Can you work these out from the model? Positions are in its coordinate system, mm. Round coordinates to 2 decimals unless told otherwise and drop trailing zeros. Loops run counter-clockwise (first coordinate to the right, second up) from the corner with the lowest first, then second, coordinate; pieces in that order, holes last. Notation, with made-up numbers: (-32.75, 82.25) -> (-23.75, 82.25) arc R25 ccw to (-23.75, 105.25) -> close; hole circle Ø8 at (1, 62.25). An arc over 180 degrees is marked (long way). Answer as a JSON object with one key per item and string values.
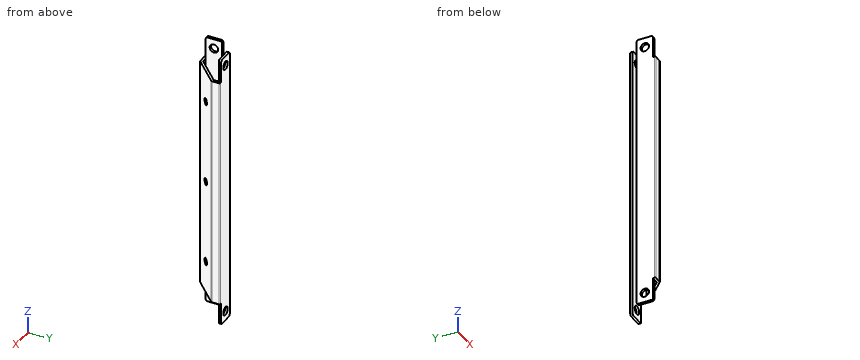
```python
from build123d import *

# Parameters (mm, degrees)
F1_DEPTH = 172.5
F3_DEPTH = 28
F4_R     = 4.25
F5_DEPTH = 25
F6_R     = 5.25
F7_DEPTH = 25
F8_R     = 5.25
F9_DEPTH = 25
F10_R    = 2
F11_R    = 0.5
F12_R    = 1


# Not quite as in the source:
# - a pattern or mirror of a feature is missing from the dataset's text; its kind, count and spacing are read off the source's solid


with BuildPart() as f1:
    # F0 (on Top) → F1 (new body, symmetric)
    with BuildSketch(Plane.XY):
        Polygon((-19.75, 3.25), (-19.75, -19.75), (-9.25, -19.75), (19.75, 9.25), (19.75, 19.75), (-3.25, 19.75), (-3.25, 16.75), (16.75, 16.75), (16.75, 10.4926406871), (-10.4926406871, -16.75), (-16.75, -16.75), (-16.75, 3.25), align=None)
    extrude(amount=F1_DEPTH, both=True)

    # F2 (on face) → F3 (cut)
    with BuildSketch(Plane.XY.offset(172.5)):
        Polygon((-10.4926406871, -16.75), (-16.75, -16.75), (-19.75, -16.75), (-19.75, -19.75), (-9.25, -19.75), (19.75, 9.25), (19.75, 19.75), (16.75, 19.75), (16.75, 16.75), (16.75, 10.4926406871), align=None)
    f3 = extrude(amount=-F3_DEPTH, mode=Mode.SUBTRACT)

    # F3_copies: F3 across plane
    add(f3.mirror(Plane(origin=(0, 0, 0), x_dir=(-1, 0, 0), z_dir=(0, 0, -1))), mode=Mode.SUBTRACT)

    # F4 (on face) → F5 (cut)
    with BuildSketch(Plane(origin=(5.25, -5.25, 0), x_dir=(0.7071067812, 0.7071067812, 0), z_dir=(0.7071067812, -0.7071067812, 0))):
        with Locations((0, 104.5)):
            Circle(F4_R)
        with Locations((0, -104.5)):
            Circle(F4_R)
        Circle(F4_R)
    extrude(amount=-F5_DEPTH, mode=Mode.SUBTRACT)

    # F6 (on face) → F7 (cut)
    with BuildSketch(Plane.YZ.offset(-16.75)):
        with Locations((-6.75, 160.5)):
            Circle(F6_R)
        with Locations((-6.75, -160.5)):
            Circle(F6_R)
    extrude(amount=-F7_DEPTH, mode=Mode.SUBTRACT)

    # F8 (on face) → F9 (cut)
    with BuildSketch(Plane.XZ.offset(-16.75)):
        with Locations((6.75, 160.5)):
            Circle(F8_R)
        with Locations((6.75, -160.5)):
            Circle(F8_R)
    extrude(amount=-F9_DEPTH, mode=Mode.SUBTRACT)

    # F10
    f10_edges = [f1.edges().sort_by_distance(p)[0] for p in [
        (-9.25, -19.75, 0),
        (19.75, 9.25, 0),
        (16.75, 18.25, 172.5),
        (-3.25, 18.25, 172.5),
        (-18.25, 3.25, 172.5),
        (-18.25, -16.75, 172.5),
        (-18.25, 3.25, -172.5),
        (-3.25, 18.25, -172.5),
        (-18.25, -16.75, -172.5),
        (16.75, 18.25, -172.5),
    ]]
    fillet(f10_edges, radius=F10_R)

    # F11
    f11_edges = [f1.edges().sort_by_distance(p)[0] for p in [
        (-10.492641, -16.75, 0),
        (16.75, 10.492641, 0),
    ]]
    fillet(f11_edges, radius=F11_R)

    # F12
    f12_edges = [f1.edges().sort_by_distance(p)[0] for p in [
        (-19.75, -19.75, 0),
        (19.75, 19.75, 0),
    ]]
    fillet(f12_edges, radius=F12_R)


solid = f1.part
```
Q1. I'm going to push flat-ended pins straight in: pin 1 (6 mm diameter, centred on x = 8, z = 80, fed in from -Y); pin 2 (2.5 mm diameter, centred on y = 17.5, z = 152.5, fed in from +X); pin 3 (1.5 mm diameter, centred on y = 19, z = 32, fed in from -X). Where does each tip first touch, or does it pass through?
Determined:
{"pin 1": "y = -5.5", "pin 2": "x = 16.75", "pin 3": "x = -3.25"}
Q2. I want a section at A-A, the plane z = -160.5. Write out the boundary of the cut face in (x, y), then the cut area to 3 significant figures.
Determined:
{"outline": "(-19.75, -16.75) -> (-16.75, -16.75) -> (-16.75, -12) -> (-19.75, -12) -> close; (-19.75, -1.5) -> (-16.75, -1.5) -> (-16.75, 3.25) -> (-19.75, 3.25) -> close; (-3.25, 16.75) -> (1.5, 16.75) -> (1.5, 19.75) -> (-3.25, 19.75) -> close; (12, 16.75) -> (16.75, 16.75) -> (16.75, 19.75) -> (12, 19.75) -> close", "area": "57.0 mm²"}
Q3. I want a section at B-B, the plane z = -32. Write out the boundary of the cut face in (x, y), then the cut area to 3 significant figures.
Determined:
{"outline": "(-19.75, -18.75) arc R1 ccw to (-18.75, -19.75) -> (-10.08, -19.75) arc R2 ccw to (-8.66, -19.16) -> (19.16, 8.66) arc R2 ccw to (19.75, 10.08) -> (19.75, 18.75) arc R1 ccw to (18.75, 19.75) -> (-3.25, 19.75) -> (-3.25, 16.75) -> (16.75, 16.75) -> (16.75, 10.7) arc R0.5 cw to (16.6, 10.35) -> (-10.35, -16.6) arc R0.5 cw to (-10.7, -16.75) -> (-16.75, -16.75) -> (-16.75, 3.25) -> (-19.75, 3.25) -> close", "area": "298 mm²"}
Q4. If I drill on L1, parallel to Z at x = -17.45, y = -6.75; L2, parallel to Z at x = 5, y = 17; L3, parallel to Y at x = -17, z = -160, over which ranges is the centre line in solid material (lowest first)? Write a range as [from, to].
Determined:
{"L1": "[-172.5, -165.75], [-155.25, 155.25], [165.75, 172.5]", "L2": "[-172.5, -165.45], [-155.55, 155.55], [165.45, 172.5]", "L3": "[-16.75, -11.98], [-1.52, 3.25]"}
